from build123d import *

# Parameters (mm, degrees)
F2_DEPTH = 25
F3_DEPTH = 0.2


with BuildPart() as f1:
    # F0 (on Front) → F1 (revolve)
    with BuildSketch(Plane.XZ):
        Polygon((-7.9381447285, 11.0953617841), (-22.9123719037, 11.0953617841), (-22.9123719037, 1.533505274), (-7.9381447285, 1.533505274), (12.6288654283, 1.533505274), (12.6288654283, 6.314433529), (-7.9381447285, 6.314433529), align=None)
    revolve(axis=Axis((12.6288654283, 0, 3.9239694015), (0, 0, -1)))

    # F2 (cut): a face of the model
    f2_faces = [f1.faces().sort_by_distance(p)[0] for p in [
        (12.6288654283, 0, 6.314433529),
    ]]
    extrude(f2_faces, amount=-F2_DEPTH, mode=Mode.SUBTRACT)

    # F3 (add): faces of the model
    f3_faces = [f1.faces().sort_by_distance(p)[0] for p in [
        (47.164844763, 0, 1.533505274),
        (34.2011335822, 0, 11.0953617841),
    ]]
    extrude(f3_faces, amount=-F3_DEPTH, dir=(0, 0, -1))


solid = f1.part
Verification items for the finished model (mm, model axes). Give positions to 0.01 mm unless a question says otherwise; leave off trailing zeros. Loops run counter-clockwise (first coordinate to the right, second up) from the corner with the lowest first, then second, coordinate; pieces in that order, holes last.
1) Draft check along X on faces 1 (the cylindrical face through (17.087, 20.078, 6.346)), 2 (the cylindrical face through (-21.27, 10.68, 6.35)), 3 (the flat face through (28, -15, 11.295)). Enter one of: pulls with the +X half, pulls with the -X half, needs draft (parallel to the pull), parting line crosses it, or undercut.
2) Sectioned sample at B-B, the plane x = 32. Enter the section's corners in (y, z), then the cut area to 3 significant figures.
3) Depth check by flat-ended pin: pin 1 Ø3 at (y, z) = (12.5, 4.5) entering from +X (3 decimals); pin 2 Ø1 at (x, z) = (-13, 2.5) entering from -Y; pin 3 Ø2 at (x, z) = (-0.5, 9.5) entering from -Y; pin 4 Ø24.5 at (x, y) = (12.63, 0) entering from +Z. Enter the tip coordinate at first touch or a pass-through.
4) Sectioned sample at C-C, the plane z = 2.75. Enter the section's corners in (x, y).
5) Sectioned sample at D-D, the plane y = -25.5. Enter the section's corners in (x, z), then the cut area to 3 significant figures.
6) Sectioned sample at A-A, the plane y = 0. Enter the section's corners in (x, z), then the cut area to 3 significant figures.
7) Thickness scan on line 1 along X through (y, z) = (1, 9); line 2 along Y through (x, z) = (19.5, 8.75); line 3 along Y through (x, z) = (14, 8.25). Record the ranges inside material, lowest first.
Answers:
1. face 1: undercut
1. face 2: parting line crosses it
1. face 3: needs draft
2. outline: (-29.8, 1.53) - (-6.91, 1.53) - (-6.91, 11.3) - (-29.8, 11.3) - close; (6.91, 1.53) - (29.8, 1.53) - (29.8, 11.3) - (6.91, 11.3) - close
2. area: 447 mm2
3. pin 1: stops at x = 46.425
3. pin 2: stops at y = -25.13
3. pin 3: stops at y = -33.41
3. pin 4: passes through
4. outline: circle Ø71.08 at (12.63, 0); hole circle Ø41.13 at (12.63, 0)
5. outline: (-12.13, 1.53) - (37.39, 1.53) - (37.39, 11.3) - (-12.13, 11.3) - close
5. area: 483 mm2
6. outline: (-22.91, 1.53) - (-7.94, 1.53) - (-7.94, 11.3) - (-22.91, 11.3) - close; (33.2, 1.53) - (48.17, 1.53) - (48.17, 11.3) - (33.2, 11.3) - close
6. area: 292 mm2
7. line 1: x = -22.9 to -7.91, 33.17 to 48.16
7. line 2: y = -34.87 to -19.39, 19.39 to 34.87
7. line 3: y = -35.51 to -20.52, 20.52 to 35.51
